Autodesk Inventor part; units mm, degrees
ref_plane "YZ Plane" through (0, 0, 0) normal (1, 0, 0) x (0, 1, 0)
ref_plane "XZ Plane" through (0, 0, 0) normal (0, 1, 0) x (-1, 0, 0)
ref_plane "XY Plane" through (0, 0, 0) normal (0, 0, 1) x (1, 0, 0)
sketch "Sketch1" plane through (0, 0, 0) normal (0, 0, 1) x (1, 0, 0)
  line L0 (0, 0) -> (3.175, 0)
  line L1 (3.175, 6.35) -> (3.175, 47.625)
  line L2 (0, 50.8) -> (0, 50.8)
  line L3 (0, 50.8) -> (0, 0)
  line L4 (0, 0) -> (50.8, 0)
  line L5 (50.8, 0) -> (50.8, 0)
  line L6 (47.625, 3.175) -> (6.35, 3.175)
  line L7 (0, 3.175) -> (0, 0)
  arc A0 (3.175, 6.35) -> (6.35, 3.175) centre (6.35, 6.35) ccw
  arc A1 (50.8, 0) -> (47.625, 3.175) centre (47.625, 0) ccw
  arc A2 (3.175, 47.625) -> (0, 50.8) centre (0, 47.625) ccw
  point P0 (3.175, 50.8)
  dimension "d0" = 3.175
  dimension "d1" = 50.8
  dimension "d2" = 3.175
  dimension "d3" = 3.175
extrude "Bracket" add sketch "Sketch1" along normal blind 190.5
sketch "Sketch2" plane through (0, 0, 0) normal (-1, 0, 0) x (0, 0, 1)
  line L0 (0, 50.8) -> (190.5, 50.8)
  line L1 (0, 50.8) -> (0, 0)
  line L2 (0, 0) -> (190.5, 0)
  line L3 (38.1, 25.4) -> (152.4, 25.4)
  dimension "d6" = 114.3
  dimension "d7" = 38.1
  dimension "d8" = 25.4
hole "Mounting Holes" at (0, 25.4, 38.1) at (0, 25.4, 152.4) direction (1, 0, 0) diameter 5.1054 end through all
sketch "Sketch3" plane through (0, 0, 0) normal (0, -1, 0) x (1, 0, 0)
  line L0 (50.8, 190.5) -> (0, 190.5)
  line L1 (0, 0) -> (0, 190.5)
  line L2 (50.8, 0) -> (50.8, 190.5)
  line L3 (37.3062, 171.45) -> (37.3063, 6.35)
  dimension "d16" = 37.3062
  dimension "d17" = 19.05
  dimension "d25" = 165.1
hole "cRIO Holes" at (37.3062, 0, 171.45) at (37.3063, 0, 6.35) direction (0, 1, 0) diameter 5.1054 end through all
properties part number "cRIO bracket"
Part model, mm, in its own coordinate system. A direction names the side the tool comes from. Coordinates: 2 decimals unless noted, no trailing zeros. Order: outer loops, then holes, each group sorted by start corner. A loop starts at its lowest first (then second) coordinate and runs counter-clockwise, first axis right, second up. Notation, with made-up numbers: (-7.5, 2) - (-3.5, 2) arc R32 ccw to (-3.5, 40) - close; hole circle Ø4 at (47.5, 49.25). An arc over 180 degrees is marked (long way). Return JSON: item names as keys, results as strings. Group by question number.
Item 1: Pull direction Y, two halves, no side cores. Call faces 3 (the face through (14, 3, 190.5)), 4 (the face through (1.61, 25.29, 149.85)), 5 (the face through (4.13, 4.08, 93.92)): pulls with the +Y half, pulls with the -Y half, needs draft (parallel to the pull), parting line crosses it, or undercut.
Item 2: Drill centre lines: probe 1 along Z at (x, y) = (2.2, 25.4); probe 2 along Y at (x, z) = (40, 159) (3 decimals); probe 3 along Y at (x, z) = (1.55, 38.1). Where is each one in solid material? Low to high. Write a range as from..to.
Item 3: Cut at C-C (x = 28). List the corners of the cut face in (y, z) (3 decimals).
Item 4: Cut at B-B (y = 25.4). List the corners of the cut face in (x, z) (3 decimals).
Item 5: Pin check, flat tips, straight feed: pin 1 (8 mm diameter, centred on x = 37.31, z = 171.45, fed in from -Y); pin 2 (2 mm diameter, centred on x = 35.5, y = 5.5, fed in from -Z); pin 3 (12 mm diameter, centred on y = 16.5, z = 94.5, fed in from +X) (3 decimals); pin 4 (20.5 mm diameter, centred on x = 21.5, z = 108, fed in from +Y) (3 decimals). Stop position of each tip, or through.
Item 6: Which spindle directions (+Z, -Z, +X, -X, +Y, -Y) get a long thin tool onto all of the face, cutting with end or side? Do faces 1 (the face through (14, 3, 0)), 2 (the face through (27, 3.175, 94)). Say none if no direction does.
Item 7: Cut at A-A (z = 38.1). List the corners of the cut face in (x, y) (3 decimals), plus the area to 3 significant figures.
Check values:
{
 "1": {"face 3": "needs draft", "face 4": "undercut", "face 5": "pulls with the +Y half"},
 "2": {"probe 1": "z = 0..35.55, 40.65..149.85, 154.95..190.5", "probe 2": "y = 0..3.175", "probe 3": "y = 0..22.85, 27.95..50.4"},
 "3": {"outline": "(0, 0) - (3.175, 0) - (3.175, 190.5) - (0, 190.5) - close"},
 "4": {"outline": "(0, 0) - (3.175, 0) - (3.175, 35.547) - (0, 35.547) - close; (0, 40.653) - (3.175, 40.653) - (3.175, 149.847) - (0, 149.847) - close; (0, 154.953) - (3.175, 154.953) - (3.175, 190.5) - (0, 190.5) - close"},
 "5": {"pin 1": "stops at y = 0", "pin 2": "passes through", "pin 3": "stops at x = 3.175", "pin 4": "stops at y = 3.175"},
 "6": {"face 1": "-Z, +X, -X, +Y, -Y", "face 2": "+Z, -Z, +X, +Y"},
 "7": {"outline": "(0, 0) - (50.8, 0) arc R3.175 ccw to (47.625, 3.175) - (6.35, 3.175) arc R3.175 cw to (3.175, 6.35) - (3.175, 22.847) - (0, 22.847) - close; (0, 27.953) - (3.175, 27.953) - (3.175, 47.625) arc R3.175 ccw to (0, 50.8) - close", "area": "294 mm2"}
}
